```python
from build123d import *

# Parameters (mm, degrees)
SKETCH1_W           = 25
SKETCH1_H           = 25
BOSS_EXTRUDE1_DEPTH = 25
SKETCH2_R           = 4
CUT_EXTRUDE1_DEPTH  = 26
SKETCH4_R           = 4.15
CUT_EXTRUDE2_DEPTH  = 26
CUT_EXTRUDE3_DEPTH  = 18
SKETCH6_R           = 1.6
CUT_EXTRUDE4_DEPTH  = 26
SKETCH7_W           = 18
SKETCH7_H           = 18
CUT_EXTRUDE5_DEPTH  = 3


with BuildPart() as part:
    # Sketch1 → Boss-Extrude1 (new body)
    with BuildSketch(Plane(origin=(0, 0, 0), x_dir=(1, 0, 0), z_dir=(0, 1, 0))):
        Rectangle(SKETCH1_W, SKETCH1_H)
    extrude(amount=BOSS_EXTRUDE1_DEPTH)

    # Sketch2 → Cut-Extrude1 (cut, through all)
    with BuildSketch(Plane.XY.offset(12.5)):
        with Locations((0, 17)):
            Circle(SKETCH2_R)
    extrude(amount=-CUT_EXTRUDE1_DEPTH, mode=Mode.SUBTRACT)

    # Sketch4 → Cut-Extrude2 (cut, through all)
    with BuildSketch(Plane(origin=(0, 25, 0), x_dir=(1, 0, 0), z_dir=(0, 1, 0))):
        with Locations(Location((0, 0, 0), (0, 0, 270))):  # turned: the seam where the file's is
            Circle(SKETCH4_R)
    extrude(amount=-CUT_EXTRUDE2_DEPTH, mode=Mode.SUBTRACT)

    # Sketch5 → Cut-Extrude3 (cut)
    with BuildSketch(Plane(origin=(0, 25, 0), x_dir=(1, 0, 0), z_dir=(0, 1, 0))):
        Polygon((-3.7, -6.408587988), (3.7, -6.408587988), (7.4, 0), (3.7, 6.408587988), (-3.7, 6.408587988), (-7.4, 0), align=None)
    extrude(amount=-CUT_EXTRUDE3_DEPTH, mode=Mode.SUBTRACT)

    # Sketch6 → Cut-Extrude4 (cut, through all)
    with BuildSketch(Plane(origin=(0, 25, 0), x_dir=(1, 0, 0), z_dir=(0, 1, 0))):
        with Locations(Location((9, -9, 0), (0, 0, 270))):  # turned: the seam where the file's is
            Circle(SKETCH6_R)
        with Locations(Location((-9, -9, 0), (0, 0, 270))):  # turned: the seam where the file's is
            Circle(SKETCH6_R)
        with Locations(Location((-9, 9, 0), (0, 0, 270))):  # turned: the seam where the file's is
            Circle(SKETCH6_R)
        with Locations(Location((9, 9, 0), (0, 0, 270))):  # turned: the seam where the file's is
            Circle(SKETCH6_R)
    extrude(amount=-CUT_EXTRUDE4_DEPTH, mode=Mode.SUBTRACT)

    # Sketch7 → Cut-Extrude5 (cut)
    with BuildSketch(Plane(origin=(0, 25, 0), x_dir=(1, 0, 0), z_dir=(0, 1, 0))):
        Rectangle(SKETCH7_W, SKETCH7_H)
    extrude(amount=-CUT_EXTRUDE5_DEPTH, mode=Mode.SUBTRACT)


solid = part.part
```
Work out the finished part from the listing and answer in its coordinate system (mm). A direction names the side the tool comes from. Give positions to 0.01 mm unless a question says otherwise; leave off trailing zeros. Loops run counter-clockwise (first coordinate to the right, second up) from the corner with the lowest first, then second, coordinate; pieces in that order, holes last. Notation, with made-up numbers: (-20.5, -38.75) - (31.5, -38.75) arc R19 ccw to (31.5, -33.75) - close; hole circle Ø1 at (36.25, 19.25). An arc over 180 degrees is marked (long way). One line per question, with ' | ' between items.
(1) A tool of negligible diameter and unlimited length cuts with its end or side. For faces 1 (the face through (-5.524, 14.605, -3.249)), 2 (the face through (-4, 17, 9)), from which of +Z, -Z, +X, -X, +Y, -Y can it reach the whole face along a straight path? Write none if from no direction.
Recorded:
face 1: +Y | face 2: +Z, -Z
(2) Each of these flat-tipped pins is pushed along its axis until it touches: pin 1 Ø2.5 at (x, z) = (-9, 9) entering from -Y; pin 2 Ø11 at (x, z) = (0, 0) entering from +Y. Where does it stop, or does it pass through?
Recorded:
pin 1: passes through | pin 2: stops at y = 7
(3) The part is cut by section A-A (y = 17). Write down the section's boundary in (x, z), then the cut area to 3 significant figures.
Recorded:
outline: (-12.5, -12.5) - (-4, -12.5) - (-4, -5.89) - (-7.4, 0) - (-4, 5.89) - (-4, 12.5) - (-12.5, 12.5) - close; (4, -12.5) - (12.5, -12.5) - (12.5, 12.5) - (4, 12.5) - (4, 5.89) - (7.4, 0) - (4, -5.89) - close; hole circle Ø3.2 at (-9, -9); hole circle Ø3.2 at (-9, 9); hole circle Ø3.2 at (9, -9); hole circle Ø3.2 at (9, 9) | area: 353 mm²
(4) Straight lines are drawn through the part: probe 1 along Z at (x, y) = (9, 5.5); probe 2 along Z at (x, y) = (5.75, 22.5); probe 3 along X at (y, z) = (3.75, 0). For each, find the intervals that lie inside material, in ascending order.
Recorded:
probe 1: z = -12.5 to -10.6, -7.4 to 7.4, 10.6 to 12.5 | probe 2: z = -12.5 to -9, 9 to 12.5 | probe 3: x = -12.5 to -4.15, 4.15 to 12.5
(5) The part is cut by section B-B (z = -10.25). Write down the section's boundary in (x, y), then the cut area to 3 significant figures.
Recorded:
outline: (-12.5, 0) - (-10, 0) - (-10, 25) - (-12.5, 25) - close; (-8, 0) - (8, 0) - (8, 25) - (-8, 25) - close; (10, 0) - (12.5, 0) - (12.5, 25) - (10, 25) - close; hole circle Ø8 at (0, 17) | area: 475 mm²
(6) The part is cut by section C-C (y = 8.75). Write down the section's boundary in (x, z), then the cut area to 3 significant figures.
Recorded:
outline: (-12.5, -12.5) - (12.5, -12.5) - (12.5, 12.5) - (-12.5, 12.5) - close; hole circle Ø3.2 at (-9, -9); hole circle Ø3.2 at (-9, 9); hole (-7.4, 0) - (-3.7, -6.41) - (3.7, -6.41) - (7.4, 0) - (3.7, 6.41) - (-3.7, 6.41) - close; hole circle Ø3.2 at (9, -9); hole circle Ø3.2 at (9, 9) | area: 451 mm²
(7) The part is cut by section D-D (x = 2.5). Write down the section's boundary in (y, z), then the cut area to 3 significant figures.
Recorded:
outline: (0, -12.5) - (13.88, -12.5) - (13.88, -6.41) - (7, -6.41) - (7, -3.31) - (0, -3.31) - close; (0, 3.31) - (7, 3.31) - (7, 6.41) - (13.88, 6.41) - (13.88, 12.5) - (0, 12.5) - close; (20.12, -12.5) - (25, -12.5) - (25, -9) - (22, -9) - (22, -6.41) - (20.12, -6.41) - close; (20.12, 6.41) - (22, 6.41) - (22, 9) - (25, 9) - (25, 12.5) - (20.12, 12.5) - close | area: 256 mm²
(8) The mould has two halves that part along X. Classify faces 3 (the face through (5.524, 14.605, 3.249)), 4 (the face through (-11, 25, 0)), 5 (the face through (-12.5, 12, 0)): +X half, -X half, draft (parallel to the pull), parting line (faces both ways), or undercut.
Recorded:
face 3: undercut | face 4: draft | face 5: -X half
